Read the model definition and answer for the solid it produces. Units are mm, in the model's axes. Face numbers are marked on the shaded views. A direction names the side the tool comes from. Coordinates: 2 decimals unless noted, no trailing zeros. Write each loop counter-clockwise with the first axis right and the second up, starting at its lowest first coordinate (ties: lowest second). Pieces come first, ordered by that corner, then holes. Notation, with made-up numbers: (28.25, 51.25) - (43.25, 51.25) arc R18 cw to (43.25, 77.25) - close; hole circle Ø2 at (27, 7). An arc over 180 degrees is marked (long way). Return JSON: item names as keys, results as strings.
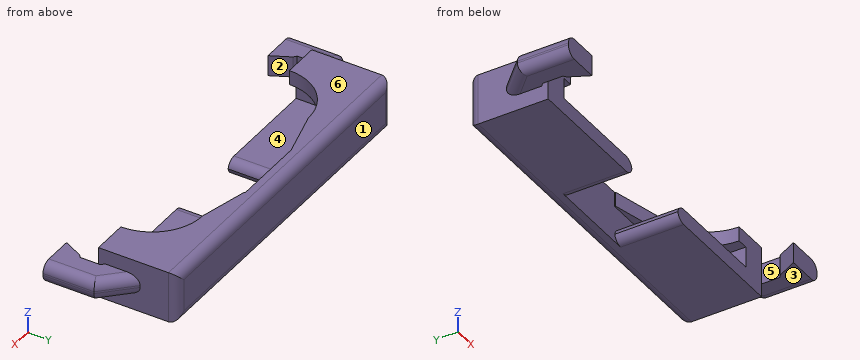
```python
from build123d import *

# Parameters (mm, degrees)
SKETCH1_W           = 54.4
SKETCH1_H           = 8.1
SKETCH1_W_2         = 46.4
SKETCH1_H_2         = 3.3
BOSS_EXTRUDE1_DEPTH = 10
SKETCH2_W           = 11.7
SKETCH2_H           = 20
CUT_EXTRUDE1_DEPTH  = 10
SKETCH3_R           = 8
CUT_EXTRUDE2_DEPTH  = 10
SKETCH4_W           = 54.4
SKETCH4_H           = 8.1
BOSS_EXTRUDE2_DEPTH = 2.6
BOSS_EXTRUDE3_DEPTH = 3.3
SKETCH2_2_W         = 11.7
SKETCH2_2_H         = 20
CUT_EXTRUDE3_DEPTH  = 20
CUT_EXTRUDE4_START  = -5
CUT_EXTRUDE4_DEPTH  = 5
SKETCH7_W           = 2.777966001
SKETCH7_H           = 4.960653573
BOSS_EXTRUDE4_DEPTH = 3.3
FILLET1_R           = 1.5
FILLET2_R           = 1.5
FILLET3_R           = 1.5
FILLET4_R           = 1.5


with BuildPart() as part:
    # Sketch1 → Boss-Extrude1 (new body)
    with BuildSketch(Plane(origin=(0, 0, 0), x_dir=(1, 0, 0), z_dir=(0, 1, 0))):
        Rectangle(SKETCH1_W, SKETCH1_H)
        with Locations((0, -0.1)):
            Rectangle(SKETCH1_W_2, SKETCH1_H_2, mode=Mode.SUBTRACT)
    extrude(amount=BOSS_EXTRUDE1_DEPTH)

    # Sketch2 → Cut-Extrude1 (cut)
    with BuildSketch(Plane.XY.offset(-1.55)):
        Rectangle(SKETCH2_W, SKETCH2_H)
    extrude(amount=-CUT_EXTRUDE1_DEPTH, mode=Mode.SUBTRACT)

    # Sketch3 → Cut-Extrude2 (cut)
    with BuildSketch(Plane(origin=(0, 0, 1.75), x_dir=(-1, 0, 0), z_dir=(0, 0, -1))):
        with Locations((-13.5, 0)):
            Circle(SKETCH3_R)
        with Locations((13.5, 0)):
            Circle(SKETCH3_R)
    extrude(amount=-CUT_EXTRUDE2_DEPTH, mode=Mode.SUBTRACT)

    # Sketch4 → Boss-Extrude2 (add)
    with BuildSketch(Plane(origin=(0, 10, 0), x_dir=(1, 0, 0), z_dir=(0, 1, 0))):
        Rectangle(SKETCH4_W, SKETCH4_H)
    extrude(amount=BOSS_EXTRUDE2_DEPTH)

    # Sketch5 → Boss-Extrude3 (add)
    with BuildSketch(Plane.XY.offset(-1.55)):
        Polygon((27.2, -6), (25.7, -6), (27.2, -3), (29.7, -0.95), (27.2, 1.001976063), (27.2, 6.6), (29.7, 4.1), (31.7, 2.1), (31.7, -6), (29.7, -6), align=None)
        Polygon((-27.2, 6.6), (-27.2, 1.001976063), (-29.7, -0.95), (-27.2, -3), (-25.7, -6), (-27.2, -6), (-29.7, -6), (-31.7, -6), (-31.7, 2.1), (-29.7, 4.1), align=None)
    extrude(amount=BOSS_EXTRUDE3_DEPTH)

    # Sketch2<2> → Cut-Extrude3 (cut)
    with BuildSketch(Plane.XY.offset(-1.55)):
        Rectangle(SKETCH2_2_W, SKETCH2_2_H)
    extrude(amount=CUT_EXTRUDE3_DEPTH, mode=Mode.SUBTRACT)

    # Sketch6 → Cut-Extrude4 (cut)
    with BuildSketch(Plane.XY.offset(4.05).offset(CUT_EXTRUDE4_START)):
        with BuildLine():
            Line((-13.5, 8), (-5.85, 10))
            Line((-5.85, 10), (5.25, 10))
            Line((5.25, 10), (13.5, 8))
            ThreePointArc((13.5, 8), (21.5, 0), (13.5, -8))
            Line((13.5, -8), (-13.5, -8))
            ThreePointArc((-13.5, -8), (-21.5, 0), (-13.5, 8))
        make_face()
    extrude(amount=CUT_EXTRUDE4_DEPTH, mode=Mode.SUBTRACT)

    # Sketch7 → Boss-Extrude4 (add)
    with BuildSketch(Plane.XY.offset(1.75)):
        with Locations((-29.069429935, -1.511833966)):
            Rectangle(SKETCH7_W, SKETCH7_H)
        with Locations((29.069429935, -1.511833966)):
            Rectangle(SKETCH7_W, SKETCH7_H)
    extrude(amount=-BOSS_EXTRUDE4_DEPTH)

    # Fillet1
    fillet1_edges = [part.edges().sort_by_distance(p)[0] for p in [
        (-27.2, 12.6, 0),
        (0, 12.6, 4.05),
        (27.2, 12.6, 0),
        (0, 12.6, -4.05),
    ]]
    fillet(fillet1_edges, radius=FILLET1_R)

    # Fillet2
    # the kernel refuses this fillet: 1.5 mm, written as the material it takes off along each edge
    with BuildSketch(Plane(origin=(5.85, 10, -1.55), x_dir=(1, 0, 0), z_dir=(0, -1, 0))) as fillet2_piece_1:
        with BuildLine():
            CenterArc((FILLET2_R, -FILLET2_R), FILLET2_R, 90, 90)
            Line((0, -FILLET2_R), (0, 0))
            Line((0, 0), (FILLET2_R, 0))
        make_face()
    extrude(amount=13.75, mode=Mode.SUBTRACT)
    with BuildSketch(Plane(origin=(5.85, 10, -4.05), x_dir=(1, 0, 0), z_dir=(0, -1, 0))) as fillet2_piece_2:
        with BuildLine():
            CenterArc((FILLET2_R, FILLET2_R), FILLET2_R, 180, 90)
            Line((0, FILLET2_R), (0, 0))
            Line((0, 0), (FILLET2_R, 0))
        make_face()
    extrude(amount=13.75, mode=Mode.SUBTRACT)

    # Fillet3
    # the kernel refuses this fillet: 1.5 mm, written as the material it takes off along each edge
    with BuildSketch(Plane(origin=(-5.85, -3.75, -1.55), x_dir=(0, 0, -1), z_dir=(0, 1, 0)), Plane(origin=(-5.85, -3.75, -4.05), x_dir=(-1, 0, 0), z_dir=(0, 1, 0))) as fillet3_piece_1:
        with BuildLine():
            CenterArc((FILLET3_R, FILLET3_R), FILLET3_R, 180, 90)
            Line((0, FILLET3_R), (0, 0))
            Line((0, 0), (FILLET3_R, 0))
        make_face()
    extrude(amount=13.75, mode=Mode.SUBTRACT)

    # Fillet4
    fillet4_edges = [part.edges().sort_by_distance(p)[0] for p in [
        (31.7, -1.95, -1.55),
        (29.45, 4.35, -1.55),
        (31.7, -1.95, 1.75),
        (29.45, 4.35, 1.75),
        (-29.45, 4.35, -1.55),
        (-31.7, -1.95, -1.55),
        (-29.45, 4.35, 1.75),
        (-31.7, -1.95, 1.75),
    ]]
    fillet(fillet4_edges, radius=FILLET4_R)


solid = part.part
```
(1) A cutting plane is placed at C-C (y = -1.25). Determine the outline of the cut face in (x, z), and give its area (3 significant figures).
Answer:
{"outline": "(-31.7, -0.05) arc R1.5 ccw to (-30.2, -1.55) - (-27.68, -1.55) - (-27.68, 1.75) - (-30.2, 1.75) arc R1.5 ccw to (-31.7, 0.25) - close; (27.68, -1.55) - (30.2, -1.55) arc R1.5 ccw to (31.7, -0.05) - (31.7, 0.25) arc R1.5 ccw to (30.2, 1.75) - (27.68, 1.75) - close", "area": "24.6 mm²"}
(2) A cutting plane is placed at D-D (z = -3.5). Determine the outline of the cut face in (x, y), and give its area (3 significant figures).
Answer:
{"outline": "(-27.2, 0) - (-6.19, 0) - (-6.19, 10) - (6.19, 10) - (6.19, 0) - (27.2, 0) - (27.2, 11.1) arc R1.5 ccw to (26.65, 12.26) - (-26.65, 12.26) arc R1.5 ccw to (-27.2, 11.1) - close", "area": "543 mm²"}
(3) A cutting plane is placed at B-B (x = 18.5). Determine the outline of the cut face in (y, z) (3 decimals).
Answer:
{"outline": "(0, -4.05) - (11.1, -4.05) arc R1.5 ccw to (12.6, -2.55) - (12.6, 2.55) arc R1.5 ccw to (11.1, 4.05) - (6.245, 4.05) - (6.245, 1.75) - (10, 1.75) - (10, -1.55) - (0, -1.55) - close"}
(4) Determine the mould class of the marked faces 1, 2 and 3 for opening direction Y: +Y half, -Y half, draft (parallel to the pull), parting line (faces both ways), or undercut.
Answer:
{"face 1": "+Y half", "face 2": "undercut", "face 3": "draft"}
(5) A cutting plane is placed at A-A (y = -4). Determine the outline of the cut face in (x, z), and give its area (3 significant figures).
Answer:
{"outline": "(-31.7, -0.05) arc R1.5 ccw to (-30.2, -1.55) - (-26.7, -1.55) - (-26.7, 1.75) - (-30.2, 1.75) arc R1.5 ccw to (-31.7, 0.25) - close; (26.7, -1.55) - (30.2, -1.55) arc R1.5 ccw to (31.7, -0.05) - (31.7, 0.25) arc R1.5 ccw to (30.2, 1.75) - (26.7, 1.75) - close", "area": "31.1 mm²"}
(6) Straight lines are drawn through the part: line 1 (Z direction, x = -23, y = 3); line 2 (Y direction, x = 20, z = 1.25); line 3 (Y direction, x = -22.5, z = 2.5). For each, find the intervals that lie inside material, in ascending order. Write a range as from..to.
Answer:
{"line 1": "-4.05..-1.55, 1.75..4.05", "line 2": "10..12.6", "line 3": "0..12.6"}
(7) Which of the six approach directions +Z, -Z, +X, -X, +Y, -Y give full straight-line access (tool end or side, diameter ignored) to the marked faces 4, 5 and 6?
Answer:
{"face 4": "-Y", "face 5": "+Z, -Z", "face 6": "+Z, +X, -X, +Y, -Y"}
(8) Flat-ended cylindrical pins translate along their axes: P1, Ø3.5, axis at y = 6, z = 0, coming from the -X side; P2, Ø2.5, axis at y = 4, z = -0.5, coming from the -X side; P3, Ø3, axis at y = 10, z = 2.5, coming from the -X side. Find the tip coordinate at first contact, or state that the pin passes through.
Answer:
{"P1": "x = -29.55", "P2": "x = -31.01", "P3": "x = -27.2"}
